For this review, take the finished solid that the model builds, in its own axes (mm). Face numbers are marked on the shaded views. A direction names the side the tool comes from. Coordinates: 2 decimals unless noted, no trailing zeros. Loops run counter-clockwise (first coordinate to the right, second up) from the corner with the lowest first, then second, coordinate; pieces in that order, holes last. Notation, with made-up numbers: M 26,-15 L 84,-15 A19 cw 84,5 Z; hole C -40,66 d2. An arc over 180 degrees is marked long. Answer as a JSON object with one key per item and string values. Group by question number.
Item 1: Add section A-A (y = 259.5). State the section outline as (x, z) points, then the cut area to 3 significant figures.
Item 2: Tool access review of the marked faces 1, 2 and 3: name each direction out of +Z, -Z, +X, -X, +Y, -Y from which nothing blocks a thin tool from reaching the whole face with its end or side.
Item 3: Insertion check: pin 1 (23 mm diameter, centred on x = 62, z = 146.5, fed in from -Y); pin 2 (12 mm diameter, centred on x = 122.5, z = 78, fed in from -Y); pin 3 (1.5 mm diameter, centred on y = 281.5, z = 152.5, fed in from +X); pin 4 (6.5 mm diameter, centred on x = 208.5, z = 150, fed in from -Y). Each pin has a flat end and moves straight along its axis. Give the tip position at first contact, or say it passes through.
Item 4: Add section B-B (x = 72.5). State the section outline as (y, z) points.
Item 5: Mouldability with a two-part tool opening along Y and no side actions: class the marked faces 4, 5, 6 and 7 as +Y half, -Y half, draft (parallel to the pull), parting line (faces both ways), or undercut.
Item 6: Add section D-D (x = 234). State the section outline as (y, z) points (3 decimals), then the cut area to 3 significant figures.
Item 7: Add section C-C (y = 359). State the section outline as (x, z) points.
Item 8: Wall thickness on L1, parallel to X at y = 216, z = 188; L2, parallel to X at y = 402.5, z = 112; L3, parallel to Y at x = 26.5, z = 109: over which ranges is each line inside the solid? List them lowest first. Write a range as from..to.
from build123d import *

# Parameters (mm, degrees)
F0_W     = 76.2
F0_H     = 406.4
F0_W_2   = 25.4
F0_H_2   = 25.4
F1_DEPTH = 203.2
F2_R     = 6.35
F3_R     = 12.7
F4_SIZE  = 12.7
F5_R     = 3.175
F6_DEPTH = 114.3


with BuildPart() as f1:
    # F0 (on Top) → F1 (new body)
    with BuildSketch(Plane.XY):
        Polygon((0, 19.00799), (19.040657, 0), (107.959343, 0), (127, 19.00799), (127, 31.727383), (118.014842, 40.727982), (127, 49.697725), (127, 215.9), (203.2, 215.9), (228.6, 215.9), (228.6, 241.3), (203.2, 241.3), (127, 241.3), (127, 407.502275), (118.014842, 416.472018), (127, 425.472617), (127, 438.19201), (107.959343, 457.2), (19.040657, 457.2), (0, 438.19201), (0, 425.472617), (8.985158, 416.472018), (0, 407.502275), (0, 49.697725), (8.985158, 40.727982), (0, 31.727383), align=None)
        with Locations((63.5, 228.6)):
            Rectangle(F0_W, F0_H, mode=Mode.SUBTRACT)
        with Locations((215.9, 203.2)):
            Rectangle(F0_W_2, F0_H_2)
        with Locations((215.9, 254)):
            Rectangle(F0_W_2, F0_H_2)
    extrude(amount=F1_DEPTH)

    # F2
    f2_edges = [f1.edges().sort_by_distance(p)[0] for p in [
        (118.014842, 416.472018, 101.6),
        (8.985158, 416.472018, 101.6),
        (8.985158, 40.727982, 101.6),
        (118.014842, 40.727982, 101.6),
    ]]
    fillet(f2_edges, radius=F2_R)

    # F3
    f3_edges = [f1.edges().sort_by_distance(p)[0] for p in [
        (127, 215.9, 101.6),
        (127, 241.3, 101.6),
    ]]
    fillet(f3_edges, radius=F3_R)

    # F4
    f4_edges = [f1.edges().sort_by_distance(p)[0] for p in [
        (228.6, 190.5, 101.6),
        (228.6, 266.7, 101.6),
    ]]
    chamfer(f4_edges, length=F4_SIZE)

    # F5 (on face) → F6 (join)
    with BuildSketch(Plane.YZ.offset(228.6)):
        with Locations((228.6, 101.6)):
            Circle(F5_R)
    extrude(amount=F6_DEPTH)


solid = f1.part
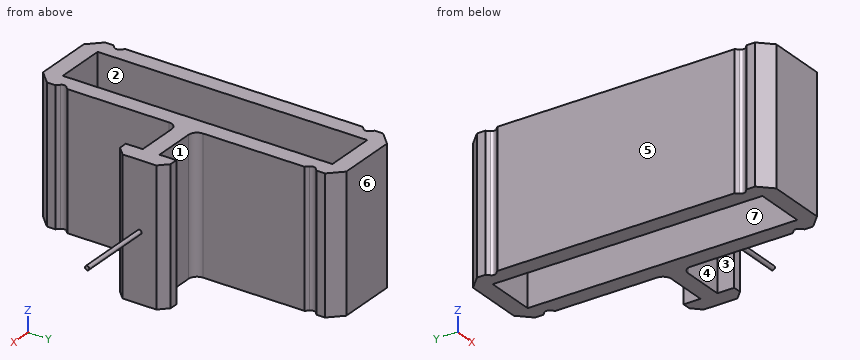
From the geometry:
{
 "1": {"outline": "M 0,0 L 25.4,0 L 25.4,203.2 L 0,203.2 Z; M 101.6,0 L 127,0 L 127,203.2 L 101.6,203.2 Z; M 203.2,0 L 223.1,0 L 223.1,203.2 L 203.2,203.2 Z", "area": "14,400 mm²"},
 "2": {"face 1": "+Z, -Z, +Y", "face 2": "+Z, -Z", "face 3": "+Z, -Z, -Y"},
 "3": {"pin 1": "stops at y = 0", "pin 2": "stops at y = 8.53", "pin 3": "stops at x = 127", "pin 4": "stops at y = 190.5"},
 "4": {"outline": "M 0,0 L 25.4,0 L 25.4,203.2 L 0,203.2 Z; M 431.8,0 L 457.2,0 L 457.2,203.2 L 431.8,203.2 Z"},
 "5": {"face 4": "-Y half", "face 5": "draft", "face 6": "+Y half", "face 7": "undercut"},
 "6": {"outline": "C 228.6,101.6 d6.35", "area": "31.7 mm²"},
 "7": {"outline": "M 0,0 L 25.4,0 L 25.4,203.2 L 0,203.2 Z; M 101.6,0 L 127,0 L 127,203.2 L 101.6,203.2 Z"},
 "8": {"L1": "x = 0..25.4, 101.6..228.6", "L2": "x = 0..25.4, 101.6..127", "L3": "y = 0..25.4, 431.8..457.2"}
}
